Read the model definition and answer for the solid it produces. Units are mm, in the model's axes. A direction names the side the tool comes from. Coordinates: 2 decimals unless noted, no trailing zeros. Use one line per item in the form item = value.
from build123d import *

# Parameters (mm, degrees)
SKETCH1_W           = 508
SKETCH1_H           = 2235.2
BOSS_EXTRUDE1_DEPTH = 317.5
CUT_EXTRUDE1_DEPTH  = 2315.084978993
SKETCH4_W           = 381
SKETCH4_H           = 2108.2
CUT_EXTRUDE2_DEPTH  = 635


with BuildPart() as part:
    # Sketch1 → Boss-Extrude1 (new, symmetric)
    with BuildSketch(Plane.XY):
        with Locations((254, 1117.6)):
            Rectangle(SKETCH1_W, SKETCH1_H)
    extrude(amount=BOSS_EXTRUDE1_DEPTH, both=True)

    # Sketch3 → Cut-Extrude1 (cut, through all)
    with BuildSketch(Plane(origin=(0, 0, 0), x_dir=(0, 0, -1), z_dir=(1, 0, 0))):
        with BuildLine():
            add(Edge.make_bspline(
                [(11.821569446, 2235.2), (53.57813934, 2051.592772393), (85.222640891, 1866.207447857), (107.434189609, 1667.229087385), (108.698878545, 1655.516041361), (111.142504459, 1632.089911804), (114.679903907, 1596.945609992), (122.036747111, 1514.906454342), (126.801961515, 1444.525721695), (134.27079546, 1303.68201965), (136.501210965, 1209.676568729), (135.828775663, 1092.031717992), (135.367512593, 1056.727910054), (134.516268219, 1021.408545813), (133.862033824, 997.858843012), (133.491664454, 986.086879756), (131.424864721, 927.264731081), (129.082951268, 880.304237017), (120.017272868, 739.710830806), (111.253713841, 646.365974306), (77.002317609, 367.455601671), (43.555969623, 183.013970543), (0, 0)],
                knots=[0, 0, 0, 0, 0.25, 0.25, 0.265625, 0.265625, 0.28125, 0.3125, 0.375, 0.375, 0.5, 0.5, 0.53125, 0.546875, 0.546875, 0.5625, 0.5625, 0.625, 0.625, 0.75, 0.75, 1, 1, 1, 1], degree=3))
            Line((0, 0), (-317.5, 0))
            Line((-317.5, 0), (-317.5, 2235.2))
            Line((-317.5, 2235.2), (11.821569446, 2235.2))
        make_face()
        with BuildLine():
            add(Edge.make_bspline(
                [(50.8, 0), (93.756857966, 183.282593988), (126.706271475, 367.938495881), (160.41784485, 647.078560023), (169.0357287, 740.484692023), (176.456558681, 857.702282187), (178.431425593, 892.902056056), (180.026988846, 928.153881246), (181.00615785, 951.666699325), (181.45337598, 963.426998719), (183.476257054, 1022.212785523), (184.41367603, 1069.223486353), (185.187938722, 1210.201925792), (182.986794075, 1304.116001508), (175.627644988, 1444.880277597), (171.716032673, 1503.509801444), (166.750196414, 1562.111566197), (164.679571807, 1585.55005263), (163.601939023, 1597.269959678), (160.24444438, 1632.408236744), (157.839846087, 1655.8074259), (134.712079658, 1866.164757361), (103.588202999, 2051.475930795), (62.441666667, 2235.2)],
                knots=[0, 0, 0, 0, 0.25, 0.25, 0.375, 0.375, 0.40625, 0.421875, 0.421875, 0.4375, 0.4375, 0.5, 0.5, 0.625, 0.625, 0.6875, 0.703125, 0.703125, 0.71875, 0.71875, 0.75, 0.75, 1, 1, 1, 1], degree=3))
            Line((62.441666667, 2235.2), (317.5, 2235.2))
            Line((317.5, 2235.2), (317.5, 0))
            Line((317.5, 0), (50.8, 0))
        make_face()
    extrude(amount=CUT_EXTRUDE1_DEPTH, mode=Mode.SUBTRACT)

    # Sketch4 → Cut-Extrude2 (cut)
    with BuildSketch(Plane.XY):
        with Locations((254, 1117.6)):
            Rectangle(SKETCH4_W, SKETCH4_H)
    extrude(amount=-CUT_EXTRUDE2_DEPTH, mode=Mode.SUBTRACT)


solid = part.part
Item 1: Find the intervals of material crossed by L1, parallel to X at y = 636, z = -119.5; L2, parallel to Y at x = 266, z = -35; L3, parallel to Z at x = 462.5, y = 1088, in increasing order.
Results below:
L1 = 0 to 63.5, 444.5 to 508
L2 = 0 to 63.5, 2171.7 to 2235.2
L3 = -184.44 to -135.73
Item 2: This flat-tipped pin is pushed along its axis until it touches: P1, Ø1.5, axis at y = 1478.5, z = -155, coming from the -X side. Where does it stop, or does it pass through?
Results below:
P1 = 0
Item 3: Which of the six approach directions +Z, -Z, +X, -X, +Y, -Y give full straight-line access (tool end or side, diameter ignored) to faces 4 (the flat face through (250, 2235.2, -37)), 5 (the flat face through (251, 2171.7, -51))?
Results below:
face_4 = +Z, -Z, +X, -X, +Y
face_5 = +Z, -Z
Item 4: For a pull along X with two mould halves and no side action, classify faces 1 (the flat face through (250, 0, -25)), 2 (the flat face through (251, 63.5, -40)), 3 (the flat face through (0, 1112, -147)) as +X half, -X half, draft (parallel to the pull), parting line (faces both ways), or undercut.
Results below:
face_1 = draft
face_2 = undercut
face_3 = -X half
Item 5: The part is cut by section A-A on z = -97. Count the separate pieces of the cut face and the enclosed holes in it, plus the area to 3 significant figures.
Results below:
separate_pieces = 4
enclosed_holes = 0
area = 79,500 mm²
